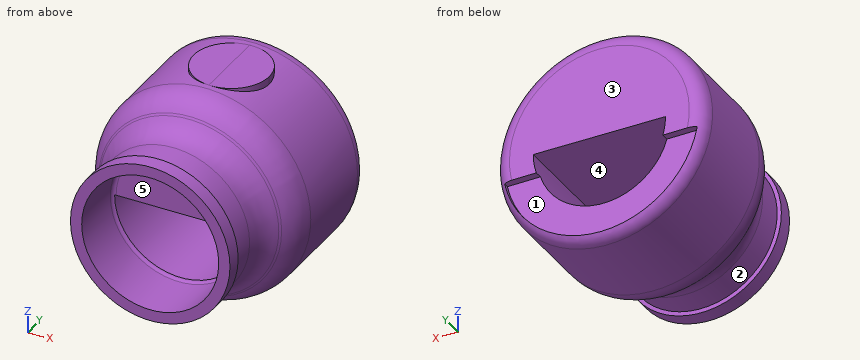
```python
from build123d import *
from build123d.topology import SkipClean

# Parameters (mm, degrees)
SKETCH10_R              = 10
BOSS_EXTRUDE1_DEPTH     = 5
CUT_EXTRUDE3_DEPTH      = 45
CUT_EXTRUDE3_DEPTH_BACK = 20
CUT_EXTRUDE5_DEPTH      = 2


with BuildPart() as part:
    # Sketch1 → Revolve1 (revolve)
    with BuildSketch(Plane.XY):
        with BuildLine():
            Line((20.9, 0), (23.871591838, 0))
            Line((23.871591838, 0), (23.871591838, 4))
            Line((23.871591838, 4), (22.9, 4.236662843))
            Line((22.9, 4.236662843), (22.9, 11.404308102))
            ThreePointArc((22.9, 11.404308102), (23.83692213, 15.63049072), (26.472123903, 19.064752533))
            Line((26.472123903, 19.064752533), (26.988320528, 19.497892931))
            ThreePointArc((26.988320528, 19.497892931), (29.623522302, 22.932154745), (30.560444431, 27.158337362))
            Line((30.560444431, 27.158337362), (30.560444431, 50))
            ThreePointArc((30.560444431, 50), (29.388871556, 52.828427125), (26.560444431, 54))
            Line((26.560444431, 54), (2.764914955, 54))
            Line((2.764914955, 54), (2.764914955, 15))
            Line((2.764914955, 15), (19.9, 15))
            ThreePointArc((19.9, 15), (20.607106781, 14.707106781), (20.9, 14))
            Line((20.9, 14), (20.9, 0))
        make_face()
    revolve(axis=Axis((2.764914955, 7.821821657, 0), (0, 1, 0)))

    # Sketch10 → Boss-Extrude1 (add)
    with SkipClean():  # the faces are left unmerged after this step: merging them gives an invalid solid
        with BuildSketch(Plane.XY.offset(27.795529476)):
            with Locations((3.346345887, 38.658337362)):
                Circle(SKETCH10_R)
        extrude(amount=-BOSS_EXTRUDE1_DEPTH)

    # Sketch11 → Cut-Extrude3 (cut, two sides: drawn at the far end of the back side and taken through both)
    with SkipClean():  # the faces are left unmerged after this step: merging them gives an invalid solid
        with BuildSketch(Plane(origin=(0, 17, 0), x_dir=(1, 0, 0), z_dir=(0, 1, 0)).offset(-CUT_EXTRUDE3_DEPTH_BACK)):
            with BuildLine():
                Line((-14.735085045, 0), (20.264914955, 0))
                ThreePointArc((20.264914955, 0), (2.764914955, 17.5), (-14.735085045, 0))
            make_face()
        extrude(amount=CUT_EXTRUDE3_DEPTH + CUT_EXTRUDE3_DEPTH_BACK, mode=Mode.SUBTRACT)

    # Sketch9 → Cut-Extrude5 (cut)
    with SkipClean():  # the faces are left unmerged after this step: merging them gives an invalid solid
        with BuildSketch(Plane(origin=(0, 54, 0), x_dir=(1, 0, 0), z_dir=(0, 1, 0))):
            with BuildLine():
                Line((-22.791277346, 4.78341249), (28.205408486, 5.364819562))
                ThreePointArc((28.205408486, 5.364819562), (2.46851135, 25.998310424), (-22.791277346, 4.78341249))
            make_face()
        extrude(amount=-CUT_EXTRUDE5_DEPTH, mode=Mode.SUBTRACT)


solid = part.part
```
Check sheet for the modelled part. Datum: model origin and axes. Units: mm. Face numbers are marked on the shaded views. A direction names the side the tool comes from. Give positions to 0.01 mm unless a question says otherwise; leave off trailing zeros. Write each loop counter-clockwise with the first axis right and the second up, starting at its lowest first coordinate (ties: lowest second). Pieces come first, ordered by that corner, then holes. Notation, with made-up numbers: (-3, 1.5) - (52, 1.5) arc R18 cw to (52, 5.5) - close; hole circle Ø11 at (1, 6). An arc over 180 degrees is marked (long way). Answer as a JSON object with one key per item and string values. Group by question number.
1) Sectioned sample at A-A (y = 46). Record the cut outline in (x, z), then the cut area to 3 significant figures.
2) Sectioned sample at C-C (y = 17). Record the cut outline in (x, z), then the cut area to 3 significant figures.
3) Release check for a two-part mould opening along X. For the marked faces 1, 2 and 3 record: pulls with the +X half, pulls with the -X half, needs draft (parallel to the pull), parting line crosses it, or undercut.
4) Depth check by flat-ended pin: P1, Ø4, axis at y = 37.5, z = 10.5, coming from the +X side; P2, Ø2, axis at x = 18.5, z = -7.5, coming from the +Y side; P3, Ø1.5, axis at x = 3, z = 15.5, coming from the -Y side. Enter the tip coordinate at first touch or a pass-through.
5) Access from +Z, -Z, +X, -X, +Y, -Y to the whole of each face (thin tool, end or side, straight path). Record for the marked faces 4 and 5.
6) Thickness scan on probe 1 along X at (y, z) = (3, 0); probe 2 along X at (y, z) = (11, 0); probe 3 along Z at (x, y) = (2.5, 32). Record the ranges inside material, lowest first. Write a range as from..to.
7) Sectioned sample at B-B (y = 10). Record the cut outline in (x, z).
Geometry results:
{
 "1": {"outline": "(-3.44, 27.09) arc R27.8 ccw (long way) to (10.14, 26.8) - (10.14, 27.8) - (-3.44, 27.8) - close; hole (-14.74, 0) arc R17.5 ccw to (20.26, 0) - close", "area": "1,950 mm^2"},
 "2": {"outline": "circle Ø43.69 at (2.76, 0); hole (-14.74, 0) arc R17.5 ccw to (20.26, 0) - close", "area": "1,020 mm^2"},
 "3": {"face 1": "undercut", "face 2": "parting line crosses it", "face 3": "needs draft"},
 "4": {"P1": "stops at x = 29.23", "P2": "stops at y = 52", "P3": "stops at y = 15"},
 "5": {"face 4": "+Y, -Y", "face 5": "-Y"},
 "6": {"probe 1": "x = -18.34..-15.37, 20.9..23.87", "probe 2": "x = -17.37..-15.37, 20.9..22.9", "probe 3": "z = -27.79..-17.5, 0..27.8"},
 "7": {"outline": "circle Ø40.27 at (2.76, 0); hole circle Ø36.27 at (2.76, 0)"}
}
